Here's the drawing with two shaded views (mm, measured from the low corner). I have some questions. Give positions to 0.01 mm unless a question says otherwise; leave off trailing zeros. Loops run counter-clockwise (first coordinate to the right, second up) from the corner with the lowest first, then second, coordinate; pieces in that order, holes last. Notation, with made-up numbers: M 21,-11 L 54,-11 A18 cw 54,6 Z; hole C 49.5,67 d8. An arc over 180 degrees is marked long. Write item = value, one per line. Start each with the question number.
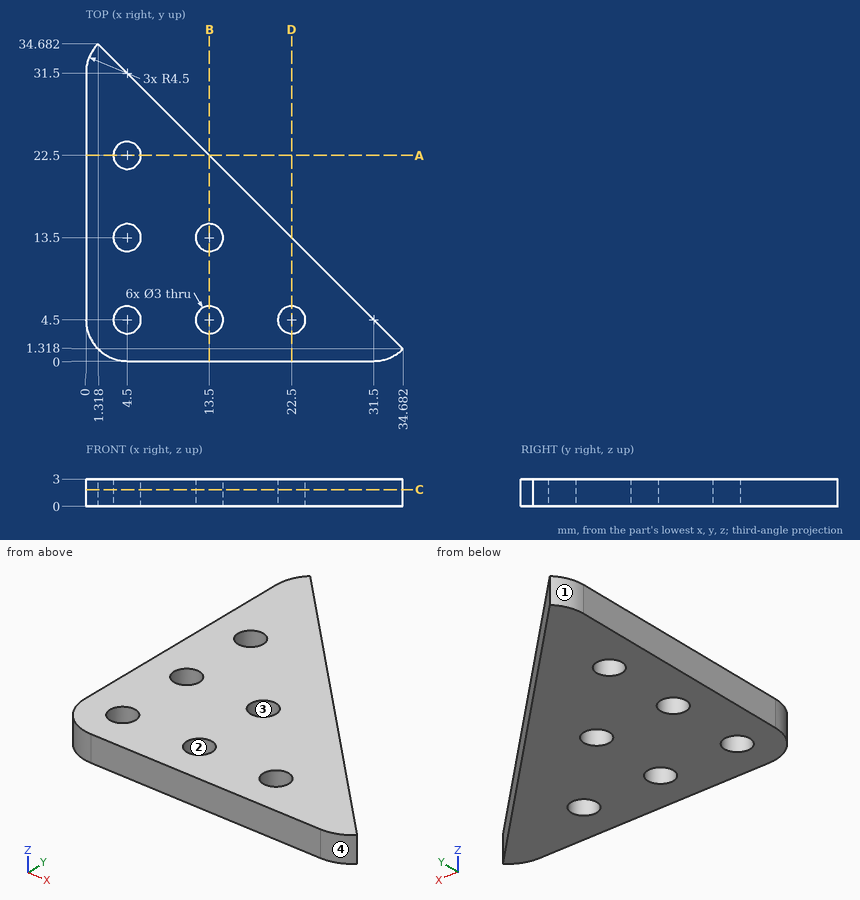
Q1. If I drill on line 1 along Y through (x, z) = (4.5, 0.9); line 2 along Y through (x, z) = (13.5, 1.8), over which ranges is the centre line in solid material (lowest first)?
Q2. If we section it at B-B, the plane x = 13.5: List the corners of the cut face in (y, z) for me, then the cut area to 3 significant figures.
Q3. If we section it at A-A, the plane y = 22.5: List the corners of the cut face in (x, z) for me.
Q4. If we section it at C-C, the plane z = 1.85: List the corners of the cut face in (x, y) for me, then the cut area to 3 significant figures.
Q5. We'd pull the mould along X, two halves only. Please class the marked faces 1, 2, 3 and 4: pulls with the +X half, pulls with the -X half, needs draft (parallel to the pull), parting line crosses it, or undercut.
Resolved:
q1.line_1 = 0 to 3, 6 to 12, 15 to 21, 24 to 31.5
q1.line_2 = 0 to 3, 6 to 12, 15 to 22.5
q2.outline = M 0,0 L 3,0 L 3,3 L 0,3 Z; M 6,0 L 12,0 L 12,3 L 6,3 Z; M 15,0 L 22.5,0 L 22.5,3 L 15,3 Z
q2.area = 49.5 mm²
q3.outline = M 0,0 L 3,0 L 3,3 L 0,3 Z; M 6,0 L 13.5,0 L 13.5,3 L 6,3 Z
q4.outline = M 0,4.5 A4.5 ccw 4.5,0 L 31.5,0 A4.5 ccw 34.68,1.32 L 1.32,34.68 A4.5 ccw 0,31.5 Z; hole C 4.5,4.5 d3; hole C 4.5,13.5 d3; hole C 4.5,22.5 d3; hole C 13.5,4.5 d3; hole C 13.5,13.5 d3; hole C 22.5,4.5 d3
q4.area = 597 mm²
q5.face_1 = pulls with the -X half
q5.face_2 = undercut
q5.face_3 = undercut
q5.face_4 = pulls with the +X half
